CAD build for the part. Positions are in the model's coordinates, mm. Face numbers are marked on the shaded views. Give positions to 0.01 mm unless a question says otherwise; leave off trailing zeros. Loops run counter-clockwise (first coordinate to the right, second up) from the corner with the lowest first, then second, coordinate; pieces in that order, holes last. Notation, with made-up numbers: (79, 82) -> (112, 82) arc R27 cw to (112, 103) -> close; hole circle Ø5 at (64, 34.25). An arc over 180 degrees is marked (long way). Use one line per item in the form item = value.
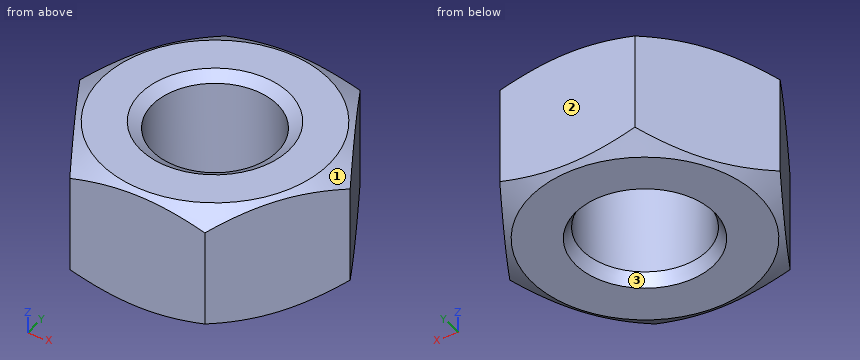
```python
from build123d import *

# Parameters (mm, degrees)
SKETCH1_R               = 4.188
BASENUT_DEPTH           = 8.4
ENDCHAMFER_SIZE         = 0.812
ENDCHAMFER_SIZE2        = 0.468808419
ENDCHAMFER_PART_2_SIZE  = 0.812
ENDCHAMFER_PART_2_SIZE2 = 0.468808419


with BuildPart() as part:
    # Sketch1 → BaseNut (new body)
    with BuildSketch(Plane.XY):
        Polygon((9.237604307, 0), (4.618802154, 8), (-4.618802154, 8), (-9.237604307, 0), (-4.618802154, -8), (4.618802154, -8), align=None)
        Circle(SKETCH1_R, mode=Mode.SUBTRACT)
    extrude(amount=-BASENUT_DEPTH)

    # Sketch2 → Double-Chamfer (revolve, cut)
    with BuildSketch(Plane(origin=(0, 0, 0), x_dir=(1, 0, 0), z_dir=(0, 1, 0))):
        Polygon((-9.237604307, 8.4), (-7.625, 8.4), (-9.237604307, 7.468962469), align=None)
        Polygon((-9.237604307, 0.931037531), (-9.237604307, 0), (-7.625, 0), align=None)
    revolve(axis=Axis((0, 0, -3.375940562), (0, 0, 1)), mode=Mode.SUBTRACT)

    # EndChamfer
    endchamfer_edges = [part.edges().sort_by_distance(p)[0] for p in [
        (-4.188, 0, -8.4),
    ]]
    endchamfer_side = [part.faces().sort_by_distance(p)[0] for p in [
        (-4.188, 0, -4.2),
    ]]
    chamfer(endchamfer_edges, length=ENDCHAMFER_SIZE, length2=ENDCHAMFER_SIZE2, reference=endchamfer_side[0])

    # EndChamfer part 2
    endchamfer_part_2_edges = [part.edges().sort_by_distance(p)[0] for p in [
        (-4.188, 0, 0),
    ]]
    endchamfer_part_2_side = [part.faces().sort_by_distance(p)[0] for p in [
        (7.409332432, 0, 0),
    ]]
    chamfer(endchamfer_part_2_edges, length=ENDCHAMFER_PART_2_SIZE, length2=ENDCHAMFER_PART_2_SIZE2, reference=endchamfer_part_2_side[0])


solid = part.part
```
1. Cut at B-B, the plane x = 0. Write the cut outline in (y, z) (1 decimal).
Result sheet:
outline = (-8, -8.2) -> (-7.6, -8.4) -> (-4.7, -8.4) -> (-4.2, -7.6) -> (-4.2, -0.5) -> (-5, 0) -> (-7.6, 0) -> (-8, -0.2) -> close; (4.2, -7.6) -> (4.7, -8.4) -> (7.6, -8.4) -> (8, -8.2) -> (8, -0.2) -> (7.6, 0) -> (5, 0) -> (4.2, -0.5) -> close
2. Drill centre lines: line 1 (Y direction, x = 0, z = -4.5); line 2 (Y direction, x = 1.5, z = -1); line 3 (X direction, y = 3, z = -1.75). Where is each one in solid material? Low to high.
Result sheet:
line_1 = -8 to -4.19, 4.19 to 8
line_2 = -8 to -3.91, 3.91 to 8
line_3 = -7.51 to -2.92, 2.92 to 7.51
3. Mould opens along Y. For the marked faces 1, 2 and 3 say: pulls with the +Y half, pulls with the -Y half, needs draft (parallel to the pull), parting line crosses it, or undercut.
Result sheet:
face_1 = parting line crosses it
face_2 = pulls with the +Y half
face_3 = undercut
4. Drop flat-ended pins along their axis: P1, Ø9.5, axis at x = 0, y = 0, coming from the +Z side; P2, Ø1.5, axis at y = 5, z = -4, coming from the -X side; P3, Ø8, axis at x = 5.5, y = -2.5, coming from the +Z side; P4, Ø5, axis at y = 4.5, z = -2, coming from the -X side. Give the stop position or say it passes through.
Result sheet:
P1 = -0.14
P2 = -6.78
P3 = 0
P4 = -8.08
5. Cut at A-A, the plane z = -1.5. Write the cut outline in (x, y).
Result sheet:
outline = (-9.24, 0) -> (-4.62, -8) -> (4.62, -8) -> (9.24, 0) -> (4.62, 8) -> (-4.62, 8) -> close; hole circle Ø8.38 at (0, 0)
